The drawing under review shows one solid part. Ordinate dimensions are in mm from its lowest x, y, z. A direction names the side the tool comes from. Give positions to 0.01 mm unless a question says otherwise; leave off trailing zeros. Order: outer loops, then holes, each group sorted by start corner. A loop starts at its lowest first (then second) coordinate and runs counter-clockwise, first axis right, second up. Notation, with made-up numbers: (-31.5, 50) -> (7.5, 50) arc R30 cw to (7.5, 78) -> close; hole circle Ø6 at (-39.75, 73). An arc over 180 degrees is marked (long way). Return JSON: item names as keys, results as strings. Group by question number.
1) To check wall thickness, follow line 1 along Z through (x, y) = (20, 24.5); line 2 along X through (y, z) = (1.05, 14); line 3 along Y through (x, z) = (18, 20.25). State the ranges of each line that lie inside material, in increasing order.
2) Add section A-A (x = 11). Give the boundary of the cut face in (y, z).
3) Add section D-D (z = 14). Give the boundary of the cut face in (x, y), then the cut area to 3 significant figures.
4) For the marked faces 1 and 2, list the 3-axis set-ups (+Z, -Z, +X, -X, +Y, -Y) from which the entire face can be reached by the end or side of a thin tool; tool diameter is ignored.
5) The part is to be moulded in two halves that separate along Z. For the marked faces 3, 4 and 5, say which applies: released by +Z, released by -Z, zero draft, split by the parting line, or undercut.
6) Add section B-B (y = 15). Give the boundary of the cut face in (x, z), then the cut area to 3 significant figures.
7) Add section C-C (z = 7). Give the boundary of the cut face in (x, y), then the cut area to 3 significant figures.
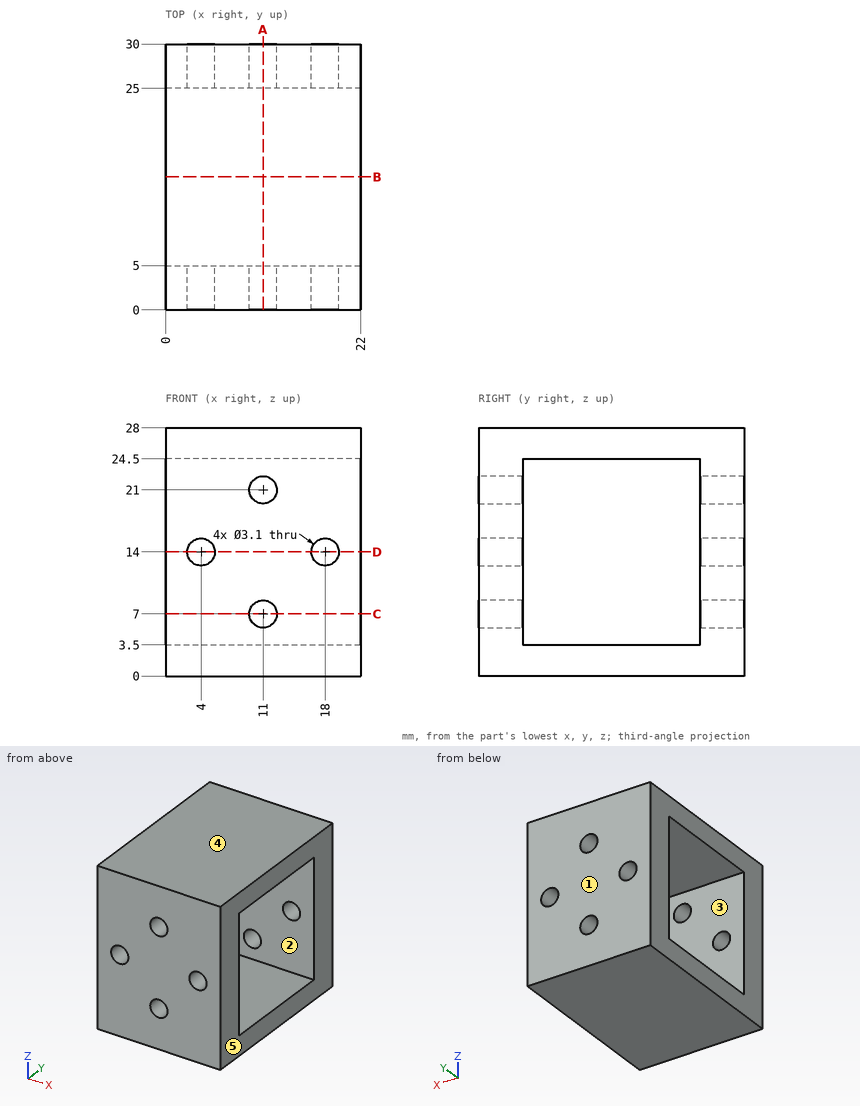
Evaluation:
{
 "1": {"line 1": "0 to 3.5, 24.5 to 28", "line 2": "0 to 2.45, 5.55 to 16.45, 19.55 to 22", "line 3": "0 to 5, 25 to 30"},
 "2": {"outline": "(0, 0) -> (30, 0) -> (30, 5.45) -> (25, 5.45) -> (25, 3.5) -> (5, 3.5) -> (5, 5.45) -> (0, 5.45) -> close; (0, 8.55) -> (5, 8.55) -> (5, 19.45) -> (0, 19.45) -> close; (0, 22.55) -> (5, 22.55) -> (5, 24.5) -> (25, 24.5) -> (25, 22.55) -> (30, 22.55) -> (30, 28) -> (0, 28) -> close; (25, 8.55) -> (30, 8.55) -> (30, 19.45) -> (25, 19.45) -> close"},
 "3": {"outline": "(0, 0) -> (2.45, 0) -> (2.45, 5) -> (0, 5) -> close; (0, 25) -> (2.45, 25) -> (2.45, 30) -> (0, 30) -> close; (5.55, 0) -> (16.45, 0) -> (16.45, 5) -> (5.55, 5) -> close; (5.55, 25) -> (16.45, 25) -> (16.45, 30) -> (5.55, 30) -> close; (19.55, 0) -> (22, 0) -> (22, 5) -> (19.55, 5) -> close; (19.55, 25) -> (22, 25) -> (22, 30) -> (19.55, 30) -> close", "area": "158 mm^2"},
 "4": {"face 1": "+Z, -Z, +X, -X, +Y", "face 2": "+X, -X"},
 "5": {"face 3": "undercut", "face 4": "released by +Z", "face 5": "zero draft"},
 "6": {"outline": "(0, 0) -> (22, 0) -> (22, 3.5) -> (0, 3.5) -> close; (0, 24.5) -> (22, 24.5) -> (22, 28) -> (0, 28) -> close", "area": "154 mm^2"},
 "7": {"outline": "(0, 0) -> (9.45, 0) -> (9.45, 5) -> (0, 5) -> close; (0, 25) -> (9.45, 25) -> (9.45, 30) -> (0, 30) -> close; (12.55, 0) -> (22, 0) -> (22, 5) -> (12.55, 5) -> close; (12.55, 25) -> (22, 25) -> (22, 30) -> (12.55, 30) -> close", "area": "189 mm^2"}
}
